Autodesk Inventor part; units mm, degrees
ref_plane "YZ Plane" through (0, 0, 0) normal (1, 0, 0) x (0, 1, 0)
ref_plane "XZ Plane" through (0, 0, 0) normal (0, 1, 0) x (-1, 0, 0)
ref_plane "XY Plane" through (0, 0, 0) normal (0, 0, 1) x (1, 0, 0)
sketch "Sketch1" plane through (0, 0, 0) normal (0, 0, 1) x (1, 0, 0)
  line L0 (0, 0) -> (0, 50.8)
  line L1 (0, 50.8) -> (3.175, 50.8)
  line L2 (3.175, 50.8) -> (3.175, 3.175)
  line L3 (3.175, 3.175) -> (35.433, 3.175)
  line L4 (35.433, 3.175) -> (35.433, 0)
  line L5 (35.433, 0) -> (0, 0)
  dimension "d0" = 50.8
  dimension "d1" = 35.433
  dimension "d2" = 3.175
  dimension "d3" = 3.175
extrude "Extrusion1" add sketch "Sketch1" along normal blind 47.625 and the other way blind 3.2004
sketch "Sketch2" plane through (0, 0, -3.2004) normal (-1, 0, 0) x (0, 0, 1)
  line L0 (0, 0) -> (0, 50.8)
  line L1 (0, 0) -> (50.8254, 0)
  line L2 (50.8254, 50.8) -> (50.8254, 0)
  line L3 (50.8254, 50.8) -> (0, 50.8)
  point P0 (3.2004, 0)
  point P1 (28.6004, 32.5438)
  dimension "d6" = 28.6004
  dimension "d8" = 32.5438
hole "Hole1" at (0, 32.5438, 25.4) direction (1, 0, 0) diameter 28.575 end through all
sketch "Sketch4" plane through (0, 0, 47.625) normal (0, -1, 0) x (1, 0, 0)
  line L0 (35.433, -50.8254) -> (0, -50.8254)
  line L1 (35.433, 0) -> (35.433, -50.8254)
  point P0 (0, -47.625)
  point P1 (13.0556, -34.9504)
  point P2 (13.0556, -9.5504)
  dimension "d29" = 15.875
  dimension "d30" = 22.3774
  dimension "d31" = 25.4
  dimension "d32" = 22.3774
hole "Hole3" at (13.0556, 0, 12.6746) at (13.0556, 0, 38.0746) direction (0, 1, 0) diameter 6.35 end through all
equation "\"d3\" = d2"
properties part number "CLB_090_ClimberMotorBearingBracket" material "Aluminum 6061"
Could you check a few things on this model? Use its own coordinates, in mm. A direction names the side the tool comes from. Round coordinates to 2 decimals unless told otherwise and drop trailing zeros. Loops run counter-clockwise (first coordinate to the right, second up) from the corner with the lowest first, then second, coordinate; pieces in that order, holes last. Notation, with made-up numbers: (76, -13.75) - (103, -13.75) arc R19 cw to (103, -7.75) - close; hole circle Ø7 at (31.25, 4). An arc over 180 degrees is marked (long way). Answer as CSV lines item,"result".
1. I want a section at B-B on y = 36.5. List the corners of the cut face in (x, z) for me (3 decimals), then the cut area to 3 significant figures.
Filled in:
outline,"(0, -3.2) - (3.175, -3.2) - (3.175, 11.671) - (0, 11.671) - close; (0, 39.129) - (3.175, 39.129) - (3.175, 47.625) - (0, 47.625) - close"
area,"74.2 mm^2"
2. I want a section at C-C on z = 37. List the corners of the cut face in (x, y) for me (3 decimals).
Filled in:
outline,"(0, 0) - (10.068, 0) - (10.068, 3.175) - (3.175, 3.175) - (3.175, 24.203) - (0, 24.203) - close; (0, 40.885) - (3.175, 40.885) - (3.175, 50.8) - (0, 50.8) - close; (16.043, 0) - (35.433, 0) - (35.433, 3.175) - (16.043, 3.175) - close"
3. For pin 1 Ø16 at (x, z) = (18, 23) entering from +Y (3 decimals); pin 2 Ø5 at (y, z) = (18, 36.5) entering from +X (3 decimals); pin 3 Ø6 at (y, z) = (41.5, 20.5) entering from -X, each with a flat end and sliding along its axis, tell me the tip position at first contact or that it passes through.
Filled in:
pin 1,"stops at y = 3.175"
pin 2,"stops at x = 3.175"
pin 3,"passes through"
4. I want a section at A-A on z = 25.4. List the corners of the cut face in (x, y) for me (3 decimals).
Filled in:
outline,"(0, 0) - (35.433, 0) - (35.433, 3.175) - (3.175, 3.175) - (3.175, 18.256) - (0, 18.256) - close; (0, 46.831) - (3.175, 46.831) - (3.175, 50.8) - (0, 50.8) - close"
5. Please list where these lines run through material, in increasing order: line 1 along Y through (x, z) = (1.65, 25.4); line 2 along Y through (x, z) = (7, 20) (3 decimals). Write a range as [from, to].
Filled in:
line 1,"y = [0, 18.26], [46.83, 50.8]"
line 2,"y = [0, 3.175]"
6. We'd pull the mould along Y, two halves only. Please class faces 1 (the face through (1.61, 22.89, 14.87)), 2 (the face through (18, 0, 22)), 3 (the face through (2, 50.8, 22)), 4 (the face through (3.175, 17, 22)): +Y half, -Y half, draft (parallel to the pull), parting line (faces both ways), or undercut.
Filled in:
face 1,"undercut"
face 2,"-Y half"
face 3,"+Y half"
face 4,"draft"
7. I want a section at D-D on x = 8.5. List the corners of the cut face in (y, z) for me (3 decimals).
Filled in:
outline,"(0, -3.2) - (3.175, -3.2) - (3.175, 47.625) - (0, 47.625) - close"
8. On a 3-axis mill with a long thin cutter (end or side, diameter ignored), from which of +Z, -Z, +X, -X, +Y, -Y can I reach the whole of each face in a straight line? I mean faces 5 (the face through (0, 19, 16)), 6 (the face through (19, 3.175, 22)). Say none if no direction works.
Filled in:
face 5,"+Z, -Z, -X, +Y, -Y"
face 6,"+Z, -Z, +X, +Y"
